Build history of the part. All positions in model axes, mm. Face numbers are marked on the shaded views. A direction names the side the tool comes from. Round coordinates to 2 decimals unless told otherwise and drop trailing zeros. Loops run counter-clockwise (first coordinate to the right, second up) from the corner with the lowest first, then second, coordinate; pieces in that order, holes last.
Autodesk Inventor part; units mm, degrees
ref_plane "YZ Plane" through (0, 0, 0) normal (1, 0, 0) x (0, 1, 0)
ref_plane "XZ Plane" through (0, 0, 0) normal (0, 1, 0) x (-1, 0, 0)
ref_plane "XY Plane" through (0, 0, 0) normal (0, 0, 1) x (1, 0, 0)
sketch "Sketch1" plane through (0, 0, 0) normal (0, 0, 1) x (1, 0, 0)
  line L0 (0, 0) -> (3, 0)
  line L1 (3, 0) -> (3, 50)
  line L2 (3, 50) -> (0, 50)
  line L3 (0, 50) -> (0, 0)
  line L4 (3, 26.5) -> (37, 26.5)
  line L5 (37, 26.5) -> (37, 23.5)
  line L6 (37, 23.5) -> (3, 23.5)
  line L7 (3, 23.5) -> (3, 26.5)
  line L8 (37, 50) -> (40, 50)
  line L9 (40, 50) -> (40, 0)
  line L10 (40, 0) -> (37, 0)
  line L11 (37, 0) -> (37, 50)
  line L12 (0, 25) -> (40, 25) construction
  dimension "d3" = 3
  dimension "d4" = 40
  dimension "d9" = 1.5
  dimension "d10" = 50
  dimension "d11" = 25
extrude "Extrusion1" add sketch "Sketch1" along normal blind 150
fillet "Fillet1" radius 0.75 4 edges at (3, 23.5, 75) (37, 23.5, 75) (37, 26.5, 75) (3, 26.5, 75)
properties part number "Arm"
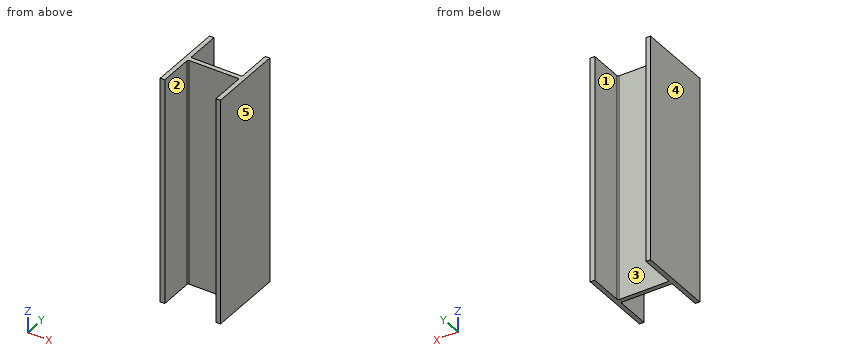
(1) Slice it at B-B on z = 28. List the corners of the cut face in (x, y), plus the area to 3 significant figures.
Responses:
outline: (0, 0) - (3, 0) - (3, 22.75) arc R0.75 cw to (3.75, 23.5) - (36.25, 23.5) arc R0.75 cw to (37, 22.75) - (37, 0) - (40, 0) - (40, 50) - (37, 50) - (37, 27.25) arc R0.75 cw to (36.25, 26.5) - (3.75, 26.5) arc R0.75 cw to (3, 27.25) - (3, 50) - (0, 50) - close
area: 402 mm2
(2) Probe line 1 (X direction, y = 43, z = 104.5); line 2 (Y direction, x = 36, z = 12). List the from-to ranges inside material, lowest first.
Responses:
line 1: x = 0 to 3, 37 to 40
line 2: y = 23.5 to 26.5
(3) Slice it at A-A on y = 29.5. List the corners of the cut face in (x, z), plus the area to 3 significant figures.
Responses:
outline: (0, 0) - (3, 0) - (3, 150) - (0, 150) - close; (37, 0) - (40, 0) - (40, 150) - (37, 150) - close
area: 900 mm2
(4) Which spindle directions (+Z, -Z, +X, -X, +Y, -Y) get a long thin tool onto all of the face, cutting with end or side? Do the marked faces 1 and 2. Say none if no direction does.
Responses:
face 1: +Z, -Z, +Y
face 2: +Z, -Z, -Y
(5) Pin check, flat tips, straight feed: P1, Ø6, axis at x = 12.5, z = 135, coming from the -Y side; P2, Ø1.5, axis at x = 32, z = 83, coming from the +Y side. Stop position of each tip, or through.
Responses:
P1: stops at y = 23.5
P2: stops at y = 26.5
(6) Slice it at C-C on x = 16. List the corners of the cut face in (y, z).
Responses:
outline: (23.5, 0) - (26.5, 0) - (26.5, 150) - (23.5, 150) - close
(7) Pull direction X, two halves, no side cores. Call the marked faces 3, 4 and 5: +X half, -X half, draft (parallel to the pull), parting line (faces both ways), or undercut.
Responses:
face 3: undercut
face 4: -X half
face 5: +X half
